```python
from build123d import *

# Parameters (mm, degrees)
SKETCH1_R           = 17.5
BOSS_EXTRUDE1_DEPTH = 2
SKETCH2_R           = 3
BOSS_EXTRUDE2_DEPTH = 5
SKETCH3_R           = 15
BOSS_EXTRUDE3_DEPTH = 16
SKETCH4_R           = 2
CUT_EXTRUDE1_DEPTH  = 5
SKETCH5_R           = 2.5
CUT_EXTRUDE2_DEPTH  = 10


with BuildPart() as part:
    # Sketch1 → Boss-Extrude1 (new body)
    with BuildSketch(Plane(origin=(0, 0, 0), x_dir=(1, 0, 0), z_dir=(0, 1, 0))):
        with Locations(Location((0, 0, 0), (0, 0, 270))):
            Circle(SKETCH1_R)
    extrude(amount=BOSS_EXTRUDE1_DEPTH)

    # Sketch2 → Boss-Extrude2 (add)
    with BuildSketch(Plane(origin=(0, 2, 0), x_dir=(1, 0, 0), z_dir=(0, 1, 0))):
        with Locations(Location((12, 0, 0), (0, 0, 270))):
            Circle(SKETCH2_R)
        with Locations(Location((0, -12, 0), (0, 0, 270))):
            Circle(SKETCH2_R)
        with Locations(Location((-12, 0, 0), (0, 0, 270))):
            Circle(SKETCH2_R)
        with Locations(Location((0, 12, 0), (0, 0, 270))):
            Circle(SKETCH2_R)
    extrude(amount=BOSS_EXTRUDE2_DEPTH)

    # Sketch3 → Boss-Extrude3 (add)
    with BuildSketch(Plane.XZ):
        with Locations(Location((0, 0, 0), (0, 0, 270))):
            Circle(SKETCH3_R)
    extrude(amount=BOSS_EXTRUDE3_DEPTH)

    # Sketch4 → Cut-Extrude1 (cut)
    with BuildSketch(Plane.XZ.offset(16)):
        with Locations(Location((-10, 0, 0), (0, 0, 270))):
            Circle(SKETCH4_R)
        with Locations(Location((0, 10, 0), (0, 0, 270))):
            Circle(SKETCH4_R)
        with Locations(Location((10, 0, 0), (0, 0, 270))):
            Circle(SKETCH4_R)
        with Locations(Location((0, -10, 0), (0, 0, 270))):
            Circle(SKETCH4_R)
    extrude(amount=-CUT_EXTRUDE1_DEPTH, mode=Mode.SUBTRACT)

    # Sketch5 → Cut-Extrude2 (cut)
    with BuildSketch(Plane(origin=(-8.121320344, 0, 8.121320344), x_dir=(0.7071067811865439, 0, 0.7071067811865512), z_dir=(-0.7071067811865512, 0, 0.7071067811865439))):
        with Locations(Location((0, -10.42298086, 0), (0, 0, 180))):
            Circle(SKETCH5_R)
    extrude(amount=CUT_EXTRUDE2_DEPTH, mode=Mode.SUBTRACT)


solid = part.part
```
The model under review builds one solid part; all positions refer to its coordinate system, in mm. A direction names the side the tool comes from. Round coordinates to 2 decimals unless told otherwise and drop trailing zeros. Loops run counter-clockwise (first coordinate to the right, second up) from the corner with the lowest first, then second, coordinate; pieces in that order, holes last. Notation, with made-up numbers: M -34,79 L 0,79 A18 cw 0,100 Z; hole C -39.5,-15.75 d3. An arc over 180 degrees is marked long. Answer as a JSON object with one key per item and string values.
(1) Take a section at B-B on z = 0. Give the boundary of the cut face in (x, y).
Resolved:
{"outline": "M -17.5,0 L -15,0 L -15,-16 L -12,-16 L -12,-11 L -8,-11 L -8,-16 L 8,-16 L 8,-11 L 12,-11 L 12,-16 L 15,-16 L 15,0 L 17.5,0 L 17.5,2 L 15,2 L 15,7 L 9,7 L 9,2 L -9,2 L -9,7 L -15,7 L -15,2 L -17.5,2 Z"}
(2) To check wall thickness, follow line 1 along X through (y, z) = (-12.7, 0); line 2 along Y through (x, z) = (-7, 1); line 3 along Y through (x, z) = (15, -4.5). State the ranges of each line that lie inside material, in increasing order.
Resolved:
{"line 1": "-15 to -12, -8 to 8, 12 to 15", "line 2": "-16 to 2", "line 3": "0 to 2"}
(3) Clearance check with flat-ended pins moving along their axes: P1, Ø2, axis at x = -12, y = -3.5, coming from the +Z side; P2, Ø12, axis at x = 4, y = -13, coming from the -Z side; P3, Ø6.5, axis at x = -10, z = 0, coming from the -Y side; P4, Ø1.5, axis at x = -2.5, y = -8.5, coming from the -Z side. State where each tip first meets the part, or that it passes through.
Resolved:
{"P1": "z = 10.2", "P2": "z = -15", "P3": "y = -16", "P4": "z = -14.9"}
(4) Take a section at C-C on y = -5.5. Give the boundary of the cut face in (x, z), and give its area (3 significant figures).
Resolved:
{"outline": "C 0,0 d30", "area": "707 mm²"}
(5) Take a section at A-A on x = 0. Give the boundary of the cut face in (y, z).
Resolved:
{"outline": "M -16,-15 L 0,-15 L 0,-17.5 L 2,-17.5 L 2,-15 L 7,-15 L 7,-9 L 2,-9 L 2,9 L 7,9 L 7,15 L 2,15 L 2,17.5 L 0,17.5 L 0,15 L -16,15 L -16,12 L -11,12 L -11,8 L -16,8 L -16,-8 L -11,-8 L -11,-12 L -16,-12 Z"}
(6) Draft analysis for pull direction Z (two halves, no side actions). For faces 1 (the cylindrical face through (0, 4, 9)), 2 (the flat face through (0, 7, 12)), 3 (the cylindrical face through (-10.648, 0.986, -13.887)), state which applies: released by +Z, released by -Z, zero draft, split by the parting line, or undercut.
Resolved:
{"face 1": "undercut", "face 2": "zero draft", "face 3": "split by the parting line"}
(7) Take a section at D-D on z = -11. Give the boundary of the cut face in (x, y), and give its area (3 significant figures).
Resolved:
{"outline": "M -13.61,0 L -10.2,0 L -10.2,-16 L -1.73,-16 L -1.73,-11 L 1.73,-11 L 1.73,-16 L 10.2,-16 L 10.2,0 L 13.61,0 L 13.61,2 L 2.83,2 L 2.83,7 L -2.83,7 L -2.83,2 L -13.61,2 Z", "area": "392 mm²"}
(8) Tool access review of faces 4 (the flat face through (-8.097, -10.458, 8.146)), 5 (the flat face through (0, -11, 10)), 6 (the flat face through (0, 2, 0)), 7 (the flat face through (-12, 7, 0)): name each direction out of +Z, -Z, +X, -X, +Y, -Y from which nothing blocks a thin tool from reaching the whole face with its end or side.
Resolved:
{"face 4": "none", "face 5": "-Y", "face 6": "+Y", "face 7": "+Z, -Z, +X, -X, +Y"}
